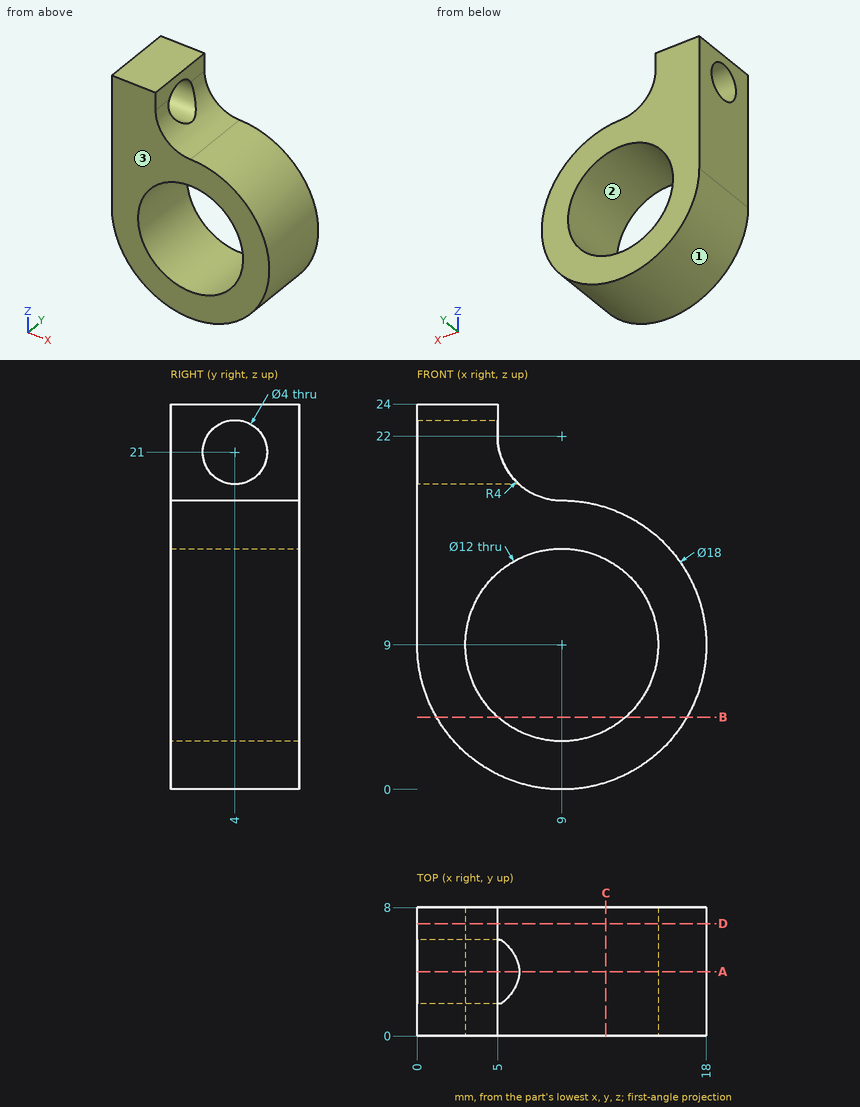
The figure shows three views and two pictorial views of one solid part (mm, origin at its lowest corner). Answer the questions. Round coordinates to 2 decimals unless told otherwise and drop trailing zeros. Order: outer loops, then holes, each group sorted by start corner. A loop starts at its lowest first (then second) coordinate and runs counter-clockwise, first axis right, second up. Notation, with made-up numbers: M -28,65.5 L -9,65.5 A14 cw -9,81.5 Z; hole C 52.5,39.25 d6. An arc over 180 degrees is marked long. Answer in a Markdown table with one row per item. Add a question column.
1) The part is cut by section B-B on z = 4.5. Determine the outline of the cut face in (x, y).
2) Consider line 1 along X through (y, z) = (0.5, 8.75); line 2 along Y through (x, z) = (3.75, 21); line 3 along Z through (x, y) = (12.5, 4.25). Determine where each line is inside the solid, lowest interval first. Write a range as from..to.
3) The part is cut by section C-C on x = 11.75. Determine the outline of the cut face in (y, z).
4) The part is cut by section A-A on y = 4. Determine the outline of the cut face in (x, z).
5) Determine the mould class of the marked faces 1, 2 and 3 for opening direction X: pulls with the +X half, pulls with the -X half, needs draft (parallel to the pull), parting line crosses it, or undercut.
6) The part is cut by section D-D on y = 7. Determine the outline of the cut face in (x, z), plus the area to 3 significant figures.
7) Flat-ended cylindrical pins translate along their axes: pin 1 Ø1 at (y, z) = (5, 23) entering from +X; pin 2 Ø7 at (x, z) = (9, 9) entering from -Y; pin 3 Ø1 at (x, y) = (11, 7) entering from -Z; pin 4 Ø2 at (y, z) = (1.5, 21.5) entering from +X. Find the tip coordinate at first contact, or state that the pin passes through.
Findings below:
| question | item | result |
|---|---|---|
| 1 | outline | M 1.21,0 L 5.03,0 L 5.03,8 L 1.21,8 Z; M 12.97,0 L 16.79,0 L 16.79,8 L 12.97,8 Z |
| 2 | line 1 | x = 0..3.01, 14.99..18 |
| 2 | line 2 | y = 0..2, 6..8 |
| 2 | line 3 | z = 0.71..4.13, 13.87..17.29 |
| 3 | outline | M 0,0.43 L 8,0.43 L 8,3.67 L 0,3.67 Z; M 0,14.33 L 8,14.33 L 8,17.57 L 0,17.57 Z |
| 4 | outline | M 0,9 A9 ccw long 9,18 A4 cw 6.35,19 L 0,19 Z; M 0,23 L 5,23 L 5,24 L 0,24 Z; hole C 9,9 d12 |
| 5 | face 1 | parting line crosses it |
| 5 | face 2 | undercut |
| 5 | face 3 | needs draft |
| 6 | outline | M 0,9 A9 ccw long 9,18 A4 cw 5,22 L 5,24 L 0,24 Z; hole C 9,9 d12 |
| 6 | area | 192 mm² |
| 7 | pin 1 | stops at x = 5 |
| 7 | pin 2 | passes through |
| 7 | pin 3 | stops at z = 0.13 |
| 7 | pin 4 | stops at x = 5.29 |
